from build123d import *

# Parameters (mm, degrees)
ESQUISSE1_W        = 21
ESQUISSE1_H        = 21
BOSS_EXTRU_1_DEPTH = 50
ESQUISSE3_W        = 21
ESQUISSE3_H        = 21
BOSS_EXTRU_2_DEPTH = 30
COQUE1_T           = -0.5
CONG_1_R           = 2


with BuildPart() as part:
    # Esquisse1 → Boss.-Extru.1 (new body)
    with BuildSketch(Plane.XY):
        Rectangle(ESQUISSE1_W, ESQUISSE1_H)
    extrude(amount=BOSS_EXTRU_1_DEPTH)

    # Esquisse3 → Boss.-Extru.2 (add)
    with BuildSketch(Plane.XZ.offset(10.5)):
        with Locations((0, 10.5)):
            Rectangle(ESQUISSE3_W, ESQUISSE3_H)
    extrude(amount=BOSS_EXTRU_2_DEPTH)

    # Coque1
    coque1_openings = [part.faces().sort_by_distance(p)[0] for p in [
        (0, 0, 50),
        (0, -40.5, 10.5),
    ]]
    offset(amount=COQUE1_T, openings=coque1_openings, kind=Kind.INTERSECTION)

    # Congé1
    cong_1_edges = [part.edges().sort_by_distance(p)[0] for p in [
        (0, 10.5, 0),
    ]]
    fillet(cong_1_edges, radius=CONG_1_R)


solid = part.part
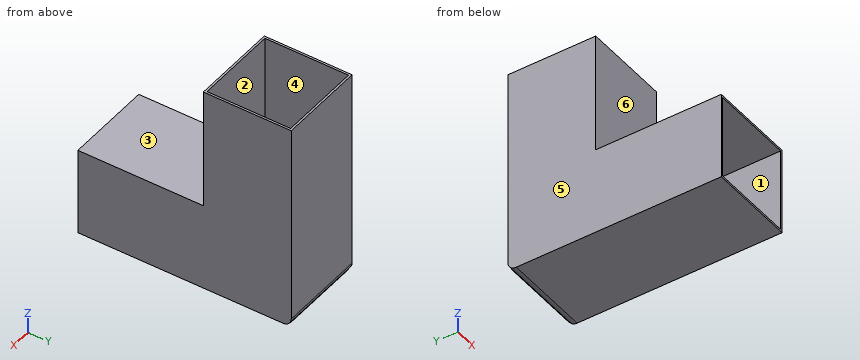
Can you work these out from the model? Positions are in its coordinate system, mm. Face numbers are marked on the shaded views. A direction names the side the tool comes from. Coordinates: 2 decimals unless noted, no trailing zeros. Write each loop counter-clockwise with the first axis right and the second up, starting at its lowest first coordinate (ties: lowest second). Pieces come first, ordered by that corner, then holes.
Q1. Imagine slicing it at D-D, the plane y = 4. List the corners of the cut face in (x, z) for me.
Results found:
outline: (-10.5, 0) - (10.5, 0) - (10.5, 50) - (10, 50) - (10, 0.5) - (-10, 0.5) - (-10, 50) - (-10.5, 50) - close
Q2. Which directions (+Z, -Z, +X, -X, +Y, -Y) give clear straight access to the entire face, cutting with the end or side of a thin tool? Please do the marked faces 1, 2 and 3.
Results found:
face 1: none
face 2: +Z
face 3: +Z, +X, -X, -Y
Q3. Imagine slicing it at C-C, the plane z = 3. List the corners of the cut face in (x, y) for me.
Results found:
outline: (-10.5, -40.5) - (-10, -40.5) - (-10, 10) - (10, 10) - (10, -40.5) - (10.5, -40.5) - (10.5, 10.5) - (-10.5, 10.5) - close
Q4. If we mould it in two halves opening along X, with no side actions, what happens to the marked faces 4, 5 and 6? For each: +X half, -X half, draft (parallel to the pull), parting line (faces both ways), or undercut.
Results found:
face 4: undercut
face 5: -X half
face 6: draft
Q5. Imagine slicing it at A-A, the plane y = -20. List the corners of the cut face in (x, z) for me, plus the area to 3 significant figures.
Results found:
outline: (-10.5, 0) - (10.5, 0) - (10.5, 21) - (-10.5, 21) - close; hole (-10, 0.5) - (10, 0.5) - (10, 20.5) - (-10, 20.5) - close
area: 41.0 mm2
Q6. Please list where these lines run through material, in increasing order: L1, parallel to Z at x = -2, y = -29; L2, parallel to X at y = -1, z = 47.
Results found:
L1: z = 0 to 0.5, 20.5 to 21
L2: x = -10.5 to -10, 10 to 10.5
Q7. For P1, Ø6.5, axis at x = 2.5, z = 29.5, coming from the -Y side; P2, Ø6.5, axis at x = 5, y = -22.5, coming from the +Z side, each with a flat end and sliding along its axis, tell me the tip position at first contact or that it passes through.
Results found:
P1: stops at y = -10.5
P2: stops at z = 21
